The drawing under review shows one solid part. Ordinate dimensions are in mm from its lowest x, y, z. A direction names the side the tool comes from. Round coordinates to 2 decimals unless told otherwise and drop trailing zeros. Write each loop counter-clockwise with the first axis right and the second up, starting at its lowest first coordinate (ties: lowest second). Pieces come first, ordered by that corner, then holes. Notation, with made-up numbers: (88.5, 20.5) -> (143.5, 20.5) arc R12 ccw to (143.5, 27.5) -> close; hole circle Ø3 at (63, -13.75). An arc over 180 degrees is marked (long way). Write item = value, one per line. Start each with the question number.
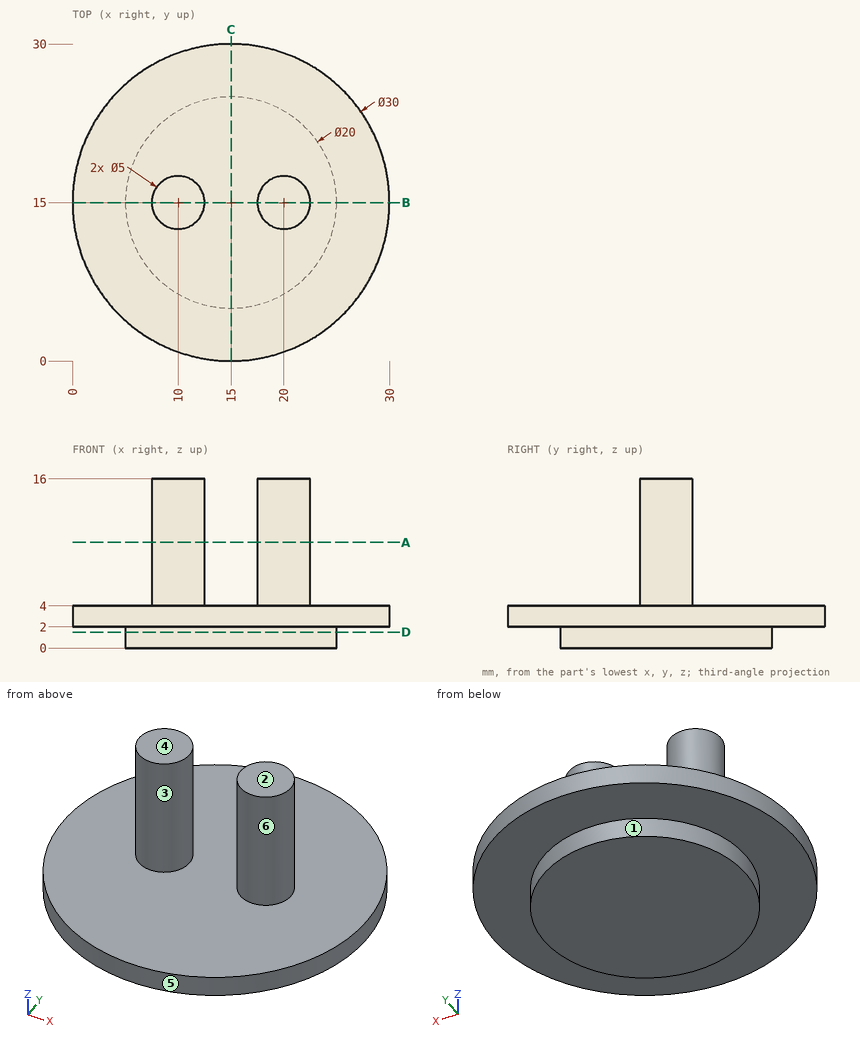
1. Machinability: for the marked faces 1, 2 and 3, which of the approach directions +Z, -Z, +X, -X, +Y, -Y give a long, thin tool a straight path to every point of the face, cutting with its end or side? Answer none if there is none.
2. Draft analysis for pull direction X (two halves, no side actions). For the marked faces 4, 5 and 6, state which applies: +X half, -X half, draft (parallel to the pull), parting line (faces both ways), or undercut.
3. Clearance check with flat-ended pins moving along their axes: pin 1 Ø6 at (x, y) = (26, 25) entering from +Z; pin 2 Ø12 at (x, y) = (25, 14) entering from -Z; pin 3 Ø4 at (x, z) = (6.5, 12.5) entering from +Y; pin 4 Ø8 at (x, z) = (23.5, 6) entering from +Y. State where each tip first meets the part, or that it passes through.
4. Consider section D-D, the plane z = 1.5. Give the boundary of the cut face in (x, y).
5. Consider section C-C, the plane x = 15. Give the boundary of the cut face in (y, z).
6. Consider section A-A, the plane z = 10. Give the boundary of the cut face in (x, y).
7. Consider section B-B, the plane y = 15. Give the boundary of the cut face in (x, z).
8. Wall thickness on L1, parallel to Z at x = 6, y = 20.75; L2, parallel to Z at x = 7.5, y = 12.75; L3, parallel to X at y = 14, z = 15.25: over which ranges is each line inside the solid? List them lowest first. Write a range as from..to.
Outcome:
q1.face_1 = -Z
q1.face_2 = +Z, +X, -X, +Y, -Y
q1.face_3 = +Z
q2.face_4 = draft
q2.face_5 = parting line
q2.face_6 = undercut
q3.pin_1 = 4
q3.pin_2 = 0
q3.pin_3 = 17
q3.pin_4 = 29.13
q4.outline = circle Ø20 at (15, 15)
q5.outline = (0, 2) -> (5, 2) -> (5, 0) -> (25, 0) -> (25, 2) -> (30, 2) -> (30, 4) -> (0, 4) -> close
q6.outline = circle Ø5 at (10, 15); circle Ø5 at (20, 15)
q7.outline = (0, 2) -> (5, 2) -> (5, 0) -> (25, 0) -> (25, 2) -> (30, 2) -> (30, 4) -> (22.5, 4) -> (22.5, 16) -> (17.5, 16) -> (17.5, 4) -> (12.5, 4) -> (12.5, 16) -> (7.5, 16) -> (7.5, 4) -> (0, 4) -> close
q8.L1 = 2..4
q8.L2 = 0..4
q8.L3 = 7.71..12.29, 17.71..22.29
